from build123d import *

# Parameters (mm, degrees)
SKETCH1_W           = 101.6
SKETCH1_H           = 127
SKETCH1_R           = 6.35
BOSS_EXTRUDE1_DEPTH = 12.0000014
SKETCH2_R           = 2.38125
CUT_EXTRUDE1_DEPTH  = 138.308557758
CIRPATTERN1_COUNT   = 6
SKETCH3_R           = 2.38125
CUT_EXTRUDE2_DEPTH  = 12.7


with BuildPart() as part:
    # Sketch1 → Boss-Extrude1 (new body)
    with BuildSketch(Plane.XY):
        with Locations((0, 63.5)):
            Rectangle(SKETCH1_W, SKETCH1_H)
        with Locations((0, 67.3749986)):
            Circle(SKETCH1_R, mode=Mode.SUBTRACT)
    extrude(amount=BOSS_EXTRUDE1_DEPTH)

    # Sketch2 → Cut-Extrude1 (cut, through all)
    with BuildSketch(Plane(origin=(0, 0, 0), x_dir=(-1, 0, 0), z_dir=(0, 0, -1))):
        with Locations((0, 107.8562486)):
            Circle(SKETCH2_R)
    cut_extrude1 = extrude(amount=-CUT_EXTRUDE1_DEPTH, mode=Mode.SUBTRACT)

    # CirPattern1: Cut-Extrude1 ×6 about axis
    cirpattern1_axis = Axis((0, 67.3749986, 0), (0, 0, 1))
    for i in range(1, CIRPATTERN1_COUNT):
        add(cut_extrude1.rotate(cirpattern1_axis, i * 360 / CIRPATTERN1_COUNT), mode=Mode.SUBTRACT)

    # Sketch3 → Cut-Extrude2 (cut)
    with BuildSketch(Plane.XZ):
        with Locations(Location((31.75, 6.0000007, 0), (0, 0, 270))):
            Circle(SKETCH3_R)
        with Locations(Location((0, 6.0000007, 0), (0, 0, 270))):
            Circle(SKETCH3_R)
        with Locations(Location((-31.75, 6.0000007, 0), (0, 0, 270))):
            Circle(SKETCH3_R)
    extrude(amount=-CUT_EXTRUDE2_DEPTH, mode=Mode.SUBTRACT)


solid = part.part
Geometry: final body of the model. Coordinates: model frame, mm. A direction names the side the tool comes from. Round coordinates to 2 decimals unless told otherwise and drop trailing zeros. Loops run counter-clockwise (first coordinate to the right, second up) from the corner with the lowest first, then second, coordinate; pieces in that order, holes last. Notation, with made-up numbers: M 20,-12 L 40,-12 A30 cw 40,23 Z; hole C 77.25,47 d1. An arc over 180 degrees is marked long. Put each result on its own line as item: value. Start each with the question number.
(1) Section query B-B (y = 69.5). Return loops of the section in (x, z), then the cut area to 3 significant figures.
(2) Contact query for flat-ended pins moving along their axis: pin 1 Ø5.5 at (x, y) = (35.06, 87.62) entering from +Z; pin 2 Ø1.4 at (x, z) = (30.5, 6) entering from -Y; pin 3 Ø4.5 at (x, y) = (35.06, 47.13) entering from +Z. Output: stop coordinate, or through.
(3) Draft query along Y for faces 1 (the face through (-0.83, 73.67, 5.92)), 2 (the face through (11, 64, 0)), 3 (the face through (0, 12.7, 6)). Return one class per face: +Y half, -Y half, draft (parallel to the pull), parting line (faces both ways), or undercut.
(4) Set-up query: faces 4 (the face through (-36.157, 45.022, 5.916)), 5 (the face through (34.11, 6.26, 6.31)). Return all of +Z, -Z, +X, -X, +Y, -Y with unobstructed straight access to the full face (end or side cutting, diameter ignored); none if empty.
(5) Section query C-C (z = 6). State how many separate pieces and enclosed holes the cut face has, then the cut area to 3 significant figures.
(6) Material intervals for line 1 along Y through (x, z) = (0, 3) (1 decimal); line 2 along Y through (x, z) = (0, 7.5) (1 decimal); line 3 along X through (y, z) = (62.5, 8.75), sorted ascending. Write a range as [from, to].
(7) Section query A-A (x = 0). Return loops of the section in (y, z) (1 decimal), then the cut area to 3 significant figures.
Findings below:
1. outline: M -50.8,0 L -5.98,0 L -5.98,12 L -50.8,12 Z; M 5.98,0 L 50.8,0 L 50.8,12 L 5.98,12 Z
1. area: 1,080 mm2
2. pin 1: stops at z = 12
2. pin 2: stops at y = 12.7
2. pin 3: passes through
3. face 1: undercut
3. face 2: draft
3. face 3: -Y half
4. face 4: +Z, -Z
4. face 5: -Y
5. separate pieces: 1
5. enclosed holes: 7
5. area: 12,500 mm2
6. line 1: y = [0, 24.5], [29.3, 61], [73.7, 105.5], [110.2, 127]
6. line 2: y = [12.7, 24.5], [29.3, 61], [73.7, 105.5], [110.2, 127]
6. line 3: x = [-50.8, -4.07], [4.07, 50.8]
7. outline: M 0,0 L 24.5,0 L 24.5,12 L 0,12 L 0,8.4 L 12.7,8.4 L 12.7,3.6 L 0,3.6 Z; M 29.3,0 L 61,0 L 61,12 L 29.3,12 Z; M 73.7,0 L 105.5,0 L 105.5,12 L 73.7,12 Z; M 110.2,0 L 127,0 L 127,12 L 110.2,12 Z
7. area: 1,200 mm2
